Here's how the part is built. I have some questions about the finished solid (model axes, mm). A direction names the side the tool comes from. Give positions to 0.01 mm unless a question says otherwise; leave off trailing zeros. Write each loop counter-clockwise with the first axis right and the second up, starting at its lowest first coordinate (ties: lowest second). Pieces come first, ordered by that corner, then holes. Notation, with made-up numbers: (21.5, 20.25) -> (29.5, 20.25) arc R14 ccw to (29.5, 31.25) -> close; hole circle Ø9 at (14, 38.25). An arc over 180 degrees is marked (long way). Answer as CSV lines item,"result". Start each with the question number.
from build123d import *

# Parameters (mm, degrees)
SALIENTE_EXTRUIR4_DEPTH  = 2
SALIENTE_EXTRUIR6_DEPTH  = 120.5
CROQUIS8_W               = 104
CROQUIS8_H               = 122.5
SALIENTE_EXTRUIR7_DEPTH  = 2
CROQUIS9_W               = 100
CROQUIS9_H               = 17
SALIENTE_EXTRUIR8_DEPTH  = 2
CROQUIS13_W              = 8.5
CROQUIS13_H              = 8.5
CROQUIS13_R              = 1.5
CROQUIS13_W_2            = 7.5
CROQUIS13_H_2            = 7.5
SALIENTE_EXTRUIR9_DEPTH  = 17
CROQUIS14_W              = 5
CROQUIS14_H              = 28
SALIENTE_EXTRUIR10_DEPTH = 122.5
CROQUIS15_W              = 5
CROQUIS15_H              = 28
SALIENTE_EXTRUIR11_DEPTH = 114
REDONDEO1_R              = 3
CORTAR_EXTRUIR1_REACH    = 153.514
CROQUIS17_W              = 5
CROQUIS17_H              = 9
CORTAR_EXTRUIR2_REACH    = 173.992
CROQUIS18_W              = 5
CROQUIS18_H              = 9
CROQUIS19_R              = 1.55
CORTAR_EXTRUIR3_DEPTH    = 11
CROQUIS20_W              = 57.7
CROQUIS20_H              = 63.5
CORTAR_EXTRUIR4_DEPTH    = 152.514025753
CROQUIS22_W              = 1.5
CROQUIS22_H              = 12
SALIENTE_EXTRUIR12_DEPTH = 30
CROQUIS26_W              = 10
CROQUIS26_H              = 5
SALIENTE_EXTRUIR14_DEPTH = 1
CROQUIS27_W              = 5
CROQUIS27_H              = 1
CORTAR_EXTRUIR8_DEPTH    = 3
CROQUIS28_W              = 1
CROQUIS28_H              = 2
CORTAR_EXTRUIR9_DEPTH    = 10
CROQUIS29_W              = 102
CROQUIS29_H              = 7.5
CORTAR_EXTRUIR11_DEPTH   = 125.5
CROQUIS30_W              = 102
CROQUIS30_H              = 19
CORTAR_EXTRUIR12_DEPTH   = 152.514025753
CROQUIS31_W              = 15
CROQUIS31_H              = 9
CORTAR_EXTRUIR13_DEPTH   = 10


with BuildPart() as part:
    # Croquis5 → Saliente-Extruir4 (new body)
    with BuildSketch(Plane.XY):
        Polygon((0, 0), (39, 0), (39, -10), (66.5, -10), (66.5, -19), (67.5, -19), (67.5, -36), (-36.5, -36), (-36.5, -19), (-35.5, -19), (-35.5, -10), (0, -10), align=None)
    extrude(amount=-SALIENTE_EXTRUIR4_DEPTH)

    # Croquis7 → Saliente-Extruir6 (add)
    with BuildSketch(Plane(origin=(0, 0, -2), x_dir=(-1, 0, 0), z_dir=(0, 0, -1))):
        Polygon((-67.5, -36), (-65.5, -36), (-65.5, -11.5), (-66.5, -11.5), (-66.5, -19), (-67.5, -19), align=None)
        Polygon((36.5, -36), (34.5, -36), (34.5, -11.5), (35.5, -11.5), (35.5, -19), (36.5, -19), align=None)
    extrude(amount=SALIENTE_EXTRUIR6_DEPTH)

    # Croquis8 → Saliente-Extruir7 (add)
    with BuildSketch(Plane.XZ.offset(36)):
        with Locations((15.5, -61.25)):
            Rectangle(CROQUIS8_W, CROQUIS8_H)
    extrude(amount=SALIENTE_EXTRUIR7_DEPTH)

    # Croquis9 → Saliente-Extruir8 (add)
    with BuildSketch(Plane(origin=(0, 0, -122.5), x_dir=(-1, 0, 0), z_dir=(0, 0, -1))):
        with Locations((-15.5, -27.5)):
            Rectangle(CROQUIS9_W, CROQUIS9_H)
    extrude(amount=-SALIENTE_EXTRUIR8_DEPTH)

    # Croquis13 → Saliente-Extruir9 (add)
    # profile 1 of 4: a face of its own
    with BuildSketch(Plane(origin=(0, -36, 0), x_dir=(1, 0, 0), z_dir=(0, 1, 0))):
        with Locations((-30.25, 6.25)):
            Rectangle(CROQUIS13_W, CROQUIS13_H)
        with Locations(Location((-30.25, 6.25, 0), (0, 0, 90))):
            Circle(CROQUIS13_R, mode=Mode.SUBTRACT)
    # profile 2 of 4: a face of its own
    with BuildSketch(Plane(origin=(0, -36, 0), x_dir=(1, 0, 0), z_dir=(0, 1, 0))):
        with Locations((-30.25, 107.25)):
            Rectangle(CROQUIS13_W, CROQUIS13_H)
        with Locations(Location((-30.25, 107.25, 0), (0, 0, 90))):
            Circle(CROQUIS13_R, mode=Mode.SUBTRACT)
    # profile 3 of 4: a face of its own
    with BuildSketch(Plane(origin=(0, -36, 0), x_dir=(1, 0, 0), z_dir=(0, 1, 0))):
        with Locations((60.75, 107.25)):
            Rectangle(CROQUIS13_W, CROQUIS13_H)
        with Locations(Location((60.75, 107.25, 0), (0, 0, 90))):
            Circle(CROQUIS13_R, mode=Mode.SUBTRACT)
    # profile 4 of 4: a face of its own
    with BuildSketch(Plane(origin=(0, -36, 0), x_dir=(1, 0, 0), z_dir=(0, 1, 0))):
        with Locations((60.75, 5.75)):
            Rectangle(CROQUIS13_W_2, CROQUIS13_H_2)
        with Locations(Location((60.75, 5.75, 0), (0, 0, 90))):
            Circle(CROQUIS13_R, mode=Mode.SUBTRACT)
    extrude(amount=SALIENTE_EXTRUIR9_DEPTH)

    # Croquis14 → Saliente-Extruir10 (add)
    with BuildSketch(Plane.XY):
        with Locations((-39, -24)):
            Rectangle(CROQUIS14_W, CROQUIS14_H)
        with Locations((70, -24)):
            Rectangle(CROQUIS14_W, CROQUIS14_H)
    extrude(amount=-SALIENTE_EXTRUIR10_DEPTH)

    # Croquis15 → Saliente-Extruir11 (add)
    with BuildSketch(Plane.ZY.offset(41.5)):
        with Locations((-125, -24)):
            Rectangle(CROQUIS15_W, CROQUIS15_H)
    extrude(amount=-SALIENTE_EXTRUIR11_DEPTH)

    # Redondeo1
    redondeo1_edges = [part.edges().sort_by_distance(p)[0] for p in [
        (-41.5, -24, 0),
        (72.5, -24, 0),
        (-41.5, -24, -127.5),
        (72.5, -24, -127.5),
    ]]
    fillet(redondeo1_edges, radius=REDONDEO1_R)

    # Croquis17 → Cortar-Extruir1 (cut, up to next)
    with BuildSketch(Plane.XY, mode=Mode.PRIVATE) as cortar_extruir1_sk1:
        with Locations((-39, -14.5)):
            Rectangle(CROQUIS17_W, CROQUIS17_H)
    cortar_extruir1_tool1 = extrude(cortar_extruir1_sk1.sketch, amount=-CORTAR_EXTRUIR1_REACH, mode=Mode.PRIVATE) & part.part
    # Croquis17 → Cortar-Extruir1 (cut, up to next)
    with BuildSketch(Plane.XY, mode=Mode.PRIVATE) as cortar_extruir1_sk2:
        with Locations((70, -14.5)):
            Rectangle(CROQUIS17_W, CROQUIS17_H)
    cortar_extruir1_tool2 = extrude(cortar_extruir1_sk2.sketch, amount=-CORTAR_EXTRUIR1_REACH, mode=Mode.PRIVATE) & part.part
    add(cortar_extruir1_tool1.solids().sort_by_distance((-39, -14.5, 0))[0], mode=Mode.SUBTRACT)
    add(cortar_extruir1_tool2.solids().sort_by_distance((70, -14.5, 0))[0], mode=Mode.SUBTRACT)

    # Croquis18 → Cortar-Extruir2 (cut, up to next)
    with BuildSketch(Plane(origin=(67.5, 0, 0), x_dir=(0, 0, -1), z_dir=(1, 0, 0)), mode=Mode.PRIVATE) as cortar_extruir2_sk1:
        with Locations((125, -14.5)):
            Rectangle(CROQUIS18_W, CROQUIS18_H)
    cortar_extruir2_tool1 = extrude(cortar_extruir2_sk1.sketch, amount=-CORTAR_EXTRUIR2_REACH, mode=Mode.PRIVATE) & part.part
    add(cortar_extruir2_tool1.solids().sort_by_distance((67.5, -14.5, -125))[0], mode=Mode.SUBTRACT)

    # Croquis19 → Cortar-Extruir3 (cut)
    with BuildSketch(Plane(origin=(0, -19, 0), x_dir=(1, 0, 0), z_dir=(0, 1, 0))):
        with Locations(Location((-38.15, 124, 0), (0, 0, 270))):
            Circle(CROQUIS19_R)
        with Locations(Location((69.15, 124, 0), (0, 0, 270))):
            Circle(CROQUIS19_R)
        with Locations(Location((-38.15, 3.5, 0), (0, 0, 270))):
            Circle(CROQUIS19_R)
        with Locations(Location((69.15, 3.5, 0), (0, 0, 270))):
            Circle(CROQUIS19_R)
    extrude(amount=-CORTAR_EXTRUIR3_DEPTH, mode=Mode.SUBTRACT)

    # Croquis20 → Cortar-Extruir4 (cut, through all)
    with BuildSketch(Plane.XZ.offset(38)):
        with Locations((15.5, -33.75)):
            Rectangle(CROQUIS20_W, CROQUIS20_H)
    extrude(amount=-CORTAR_EXTRUIR4_DEPTH, mode=Mode.SUBTRACT)

    # Croquis22 → Saliente-Extruir12 (add)
    with BuildSketch(Plane(origin=(0, 0, -2), x_dir=(-1, 0, 0), z_dir=(0, 0, -1))):
        with Locations((-45.1, -30)):
            Rectangle(CROQUIS22_W, CROQUIS22_H)
        with Locations((14.1, -30)):
            Rectangle(CROQUIS22_W, CROQUIS22_H)
    extrude(amount=SALIENTE_EXTRUIR12_DEPTH)

    # Croquis26 → Saliente-Extruir14 (add)
    with BuildSketch(Plane(origin=(0, -36, 0), x_dir=(1, 0, 0), z_dir=(0, 1, 0))):
        with Locations((15.5, 68)):
            Rectangle(CROQUIS26_W, CROQUIS26_H)
    extrude(amount=SALIENTE_EXTRUIR14_DEPTH)

    # Croquis27 → Cortar-Extruir8 (cut)
    with BuildSketch(Plane.XY.offset(-65.5)):
        with Locations((15.5, -36.5)):
            Rectangle(CROQUIS27_W, CROQUIS27_H)
    extrude(amount=-CORTAR_EXTRUIR8_DEPTH, mode=Mode.SUBTRACT)

    # Croquis28 → Cortar-Extruir9 (cut)
    with BuildSketch(Plane.XY):
        with Locations((43.85, -37)):
            Rectangle(CROQUIS28_W, CROQUIS28_H)
        with Locations((-12.85, -37)):
            Rectangle(CROQUIS28_W, CROQUIS28_H)
    extrude(amount=-CORTAR_EXTRUIR9_DEPTH, mode=Mode.SUBTRACT)

    # Croquis29 → Cortar-Extruir11 (cut)
    with BuildSketch(Plane(origin=(0, 0, -127.5), x_dir=(-1, 0, 0), z_dir=(0, 0, -1))):
        with Locations((-15.5, -15.25)):
            Rectangle(CROQUIS29_W, CROQUIS29_H)
    extrude(amount=-CORTAR_EXTRUIR11_DEPTH, mode=Mode.SUBTRACT)

    # Croquis30 → Cortar-Extruir12 (cut, through all)
    with BuildSketch(Plane.XY):
        with Locations((15.5, -9.5)):
            Rectangle(CROQUIS30_W, CROQUIS30_H)
    extrude(amount=-CORTAR_EXTRUIR12_DEPTH, mode=Mode.SUBTRACT)

    # Croquis31 → Cortar-Extruir13 (cut)
    with BuildSketch(Plane(origin=(72.5, 0, 0), x_dir=(0, 0, -1), z_dir=(1, 0, 0))):
        with Locations((65, -30.5)):
            Rectangle(CROQUIS31_W, CROQUIS31_H)
    extrude(amount=-CORTAR_EXTRUIR13_DEPTH, mode=Mode.SUBTRACT)


solid = part.part
Item 1: If we section it at D-D (y = -28): State how many separate pieces and enclosed holes the cut face has, and give its area (3 significant figures).
Item 2: We'd pull the mould along Y, two halves only. Please class faces 1 (the face through (15, -38, -79)), 2 (the face through (69, -26, -65)), 3 (the face through (57, -28, -6)): released by +Y, released by -Y, zero draft, split by the parting line, or undercut.
Item 3: If I drill on line 1 (Z direction, x = 69.15, y = -24); line 2 (X direction, y = -22.75, z = -3.5); line 3 (Z direction, x = 1.5, y = -23.75), over which ranges is the centre line in solid material (lowest first)? Write a range as [from, to].
Item 4: If we section it at B-B (x = -22.5): Please give me the cut outline in (y, z).
Item 5: I'm going to push flat-ended pins straight in: pin 1 (8 mm diameter, centred on x = -16.5, z = -69, fed in from +Y); pin 2 (12 mm diameter, centred on x = 45.5, z = -21.5, fed in from +Y). Where does each tip first touch, or does it pass through?
Item 6: For faces 4 (the face through (15.1, -37.2, -65.5)), 5 (the face through (-35, -19, -78)), 6 (the face through (-31.26, -27.62, -5.14)), which set-ups out of +Z, -Z, +X, -X, +Y, -Y let a thin tool reach every point of the face, with its end or its side?
Item 7: If we section it at A-A (x = 4.5): Please give me the cut outline in (y, z), and give its area (3 significant figures).
Item 8: If we section it at C-C (z = -113): Please give me the cut outline in (x, y).
Final values:
1,separate pieces,"2"
1,enclosed holes,"8"
1,area,"2,880 mm2"
2,face 1,"released by -Y"
2,face 2,"undercut"
2,face 3,"zero draft"
3,line 1,"[-127.5, -125.55], [-122.45, -5.05], [-1.95, 0]"
3,line 2,"[-41.5, -39.7], [-36.6, -26], [57, 64.5], [65.5, 67.6], [70.7, 72.5]"
3,line 3,"[-127.5, -120.5], [-2, 0]"
4,outline,"(-38, -127.5) -> (-19, -127.5) -> (-19, -120.5) -> (-36, -120.5) -> (-36, -2) -> (-19, -2) -> (-19, 0) -> (-38, 0) -> close"
5,pin 1,"y = -36"
5,pin 2,"y = -24"
6,face 4,"+Y, -Y"
6,face 5,"+Z, -Z, +X, -X, +Y"
6,face 6,"+Y"
7,outline,"(-38, -127.5) -> (-19, -127.5) -> (-19, -120.5) -> (-36, -120.5) -> (-36, -65.5) -> (-38, -65.5) -> close; (-38, -2) -> (-19, -2) -> (-19, 0) -> (-38, 0) -> close"
7,area,"281 mm2"
8,outline,"(-41.5, -38) -> (72.5, -38) -> (72.5, -19) -> (65.5, -19) -> (65.5, -36) -> (-34.5, -36) -> (-34.5, -19) -> (-41.5, -19) -> close"
